Autodesk Inventor part; units mm, degrees
ref_plane "YZ Plane" through (0, 0, 0) normal (1, 0, 0) x (0, 1, 0)
ref_plane "XZ Plane" through (0, 0, 0) normal (0, 1, 0) x (-1, 0, 0)
ref_plane "XY Plane" through (0, 0, 0) normal (0, 0, 1) x (1, 0, 0)
sketch "Sketch1" plane through (0, 0, 0) normal (0, 1, 0) x (-1, 0, 0)
  circle A0 centre (0, 0) radius 3
  circle A1 centre (0, 0) radius 5
  dimension "d0" = 6
  dimension "d1" = 10
extrude "Extrusion1" add sketch "Sketch1" along normal blind 3
sketch "Sketch2" plane through (0, 3, 0) normal (0, 1, 0) x (1, 0, 0)
  circle A0 centre (0, 0) radius 5
  circle A1 centre (0, 0) radius 3
  circle A2 centre (0, 0) radius 3.5
  circle A3 centre (0, 0) radius 4.5
  dimension "d4" = 7
  dimension "d5" = 9
extrude "Extrusion2" cut sketch "Sketch2" against normal blind 0.1 contours A3
sketch "Sketch3" plane through (0, 0, 0) normal (0, -1, 0) x (1, 0, 0)
  circle A0 centre (0, 0) radius 3.5
  circle A1 centre (0, 0) radius 4.5
extrude "Extrusion3" cut sketch "Sketch3" against normal blind 0.1
properties part number "bearing_6_10_3"
CAD build for the part. Positions are in the model's coordinates, mm. A direction names the side the tool comes from. Coordinates: 2 decimals unless noted, no trailing zeros. Write each loop counter-clockwise with the first axis right and the second up, starting at its lowest first coordinate (ties: lowest second). Pieces come first, ordered by that corner, then holes. Notation, with made-up numbers: (30, 47) -> (70, 47) arc R11 ccw to (70, 51) -> close; hole circle Ø2 at (-34.75, -35.5). An arc over 180 degrees is marked (long way). Return JSON: item names as keys, results as strings. Group by question number.
Q1. Cut at C-C, the plane y = 1.1. Give the cut face in (x, z).
Q2. Flat gauge pin, fed straight in: pin 1 (1.5 mm diameter, centred on x = 2, y = 1.5, fed in from +Z). Where does the tip first touch, or does it go through?
Q3. Cut at A-A, the plane z = 0. Give the cut face in (x, y), then the cut area to 3 significant figures.
Q4. Which spindle directions (+Z, -Z, +X, -X, +Y, -Y) get a long thin tool onto all of the face, cutting with end or side? Do faces 1 (the face through (0, 0.1, -4)), 2 (the face through (-3, 3, 1)), 3 (the face through (0, 2.9, 4)). Say none if no direction does.
Q5. Cut at B-B, the plane x = 0. Give the cut face in (y, z).
Q6. Drill centre lines: line 1 (Z direction, x = 0, y = 0.05); line 2 (Z direction, x = 0, y = 0.9); line 3 (X direction, y = 0.5, z = -0.75). Where is each one in solid material? Low to high.
Q7. Pull direction X, two halves, no side cores. Call faces 4 (the face through (3, 1, 0)), 5 (the face through (-3, 0, 1)), 6 (the face through (1.08, 1.48, 4.88)): released by +X, released by -X, zero draft, split by the parting line, or undercut.
Returned:
{
 "1": {"outline": "circle Ø10 at (0, 0); hole circle Ø6 at (0, 0)"},
 "2": {"pin 1": "stops at z = 4.84"},
 "3": {"outline": "(-5, 0) -> (-4.5, 0) -> (-4.5, 0.1) -> (-3.5, 0.1) -> (-3.5, 0) -> (-3, 0) -> (-3, 3) -> (-3.5, 3) -> (-3.5, 2.9) -> (-4.5, 2.9) -> (-4.5, 3) -> (-5, 3) -> close; (3, 0) -> (3.5, 0) -> (3.5, 0.1) -> (4.5, 0.1) -> (4.5, 0) -> (5, 0) -> (5, 3) -> (4.5, 3) -> (4.5, 2.9) -> (3.5, 2.9) -> (3.5, 3) -> (3, 3) -> close", "area": "11.6 mm2"},
 "4": {"face 1": "-Y", "face 2": "+Z, -Z, +X, -X, +Y", "face 3": "+Y"},
 "5": {"outline": "(0, -5) -> (3, -5) -> (3, -4.5) -> (2.9, -4.5) -> (2.9, -3.5) -> (3, -3.5) -> (3, -3) -> (0, -3) -> (0, -3.5) -> (0.1, -3.5) -> (0.1, -4.5) -> (0, -4.5) -> close; (0, 3) -> (3, 3) -> (3, 3.5) -> (2.9, 3.5) -> (2.9, 4.5) -> (3, 4.5) -> (3, 5) -> (0, 5) -> (0, 4.5) -> (0.1, 4.5) -> (0.1, 3.5) -> (0, 3.5) -> close"},
 "6": {"line 1": "z = -5 to -4.5, -3.5 to -3, 3 to 3.5, 4.5 to 5", "line 2": "z = -5 to -3, 3 to 5", "line 3": "x = -4.94 to -2.9, 2.9 to 4.94"},
 "7": {"face 4": "undercut", "face 5": "zero draft", "face 6": "split by the parting line"}
}
